from build123d import *

# Parameters (mm, degrees)
SKETCH1_R               = 1.5
BOSS_EXTRUDE1_DEPTH     = 3.5
SKETCH2_R               = 6.4
BOSS_EXTRUDE2_DEPTH     = 25
SKETCH3_R               = 2.8
CUT_EXTRUDE1_DEPTH      = 29.5
SKETCH6_R               = 9.569614172
CUT_EXTRUDE6_DEPTH      = 7.5
SKETCH7_R               = 17.775779512
SKETCH7_R_2             = 6.25
CUT_EXTRUDE7_DEPTH      = 7.5
SKETCH8_R               = 1
CUT_EXTRUDE8_DEPTH      = 4.5
SKETCH9_R               = 2
CUT_EXTRUDE9_DEPTH      = 13
CUT_EXTRUDE9_DEPTH_BACK = 1


with BuildPart() as part:
    # Sketch1 → Boss-Extrude1 (new body)
    with BuildSketch(Plane.XY):
        with BuildLine():
            Line((-14.730127019, -3.5044428), (-4.330127019, 14.508885599))
            ThreePointArc((-4.330127019, 14.508885599), (0, 17.008885599), (4.330127019, 14.508885599))
            Line((4.330127019, 14.508885599), (14.730127019, -3.5044428))
            ThreePointArc((14.730127019, -3.5044428), (14.730127019, -8.5044428), (10.4, -11.0044428))
            Line((10.4, -11.0044428), (-10.4, -11.0044428))
            ThreePointArc((-10.4, -11.0044428), (-14.730127019, -8.5044428), (-14.730127019, -3.5044428))
        make_face()
        with Locations((0, 12.008885599)):
            Circle(SKETCH1_R, mode=Mode.SUBTRACT)
        with Locations((-10.4, -6.0044428)):
            Circle(SKETCH1_R, mode=Mode.SUBTRACT)
        with Locations((10.4, -6.0044428)):
            Circle(SKETCH1_R, mode=Mode.SUBTRACT)
    extrude(amount=BOSS_EXTRUDE1_DEPTH)

    # Sketch2 → Boss-Extrude2 (add)
    with BuildSketch(Plane.XY.offset(3.5)):
        Circle(SKETCH2_R)
    extrude(amount=BOSS_EXTRUDE2_DEPTH)

    # Sketch3 → Cut-Extrude1 (cut, through all)
    with BuildSketch(Plane.XY.offset(28.5)):
        Circle(SKETCH3_R)
    extrude(amount=-CUT_EXTRUDE1_DEPTH, mode=Mode.SUBTRACT)

    # Sketch6 → Cut-Extrude6 (cut)
    with BuildSketch(Plane.XY.offset(26.5)):
        Circle(SKETCH6_R)
        Polygon((7, 0), (4.452808103, 0.65), (4.435733208, 0.757806641), (6.657395614, 2.163118961), (4.034011116, 1.994180112), (3.984457842, 2.091433888), (5.663118961, 4.114496766), (3.220337014, 3.14315598), (3.14315598, 3.220337014), (4.114496766, 5.663118961), (2.091433888, 3.984457842), (1.994180112, 4.034011116), (2.163118961, 6.657395614), (0.757806641, 4.435733208), (0.65, 4.452808103), (0, 7), (-0.65, 4.452808103), (-0.757806641, 4.435733208), (-2.163118961, 6.657395614), (-1.994180112, 4.034011116), (-2.091433888, 3.984457842), (-4.114496766, 5.663118961), (-3.14315598, 3.220337014), (-3.220337014, 3.14315598), (-5.663118961, 4.114496766), (-3.984457842, 2.091433888), (-4.034011116, 1.994180112), (-6.657395614, 2.163118961), (-4.435733208, 0.757806641), (-4.452808103, 0.65), (-7, 0), (-4.452808103, -0.65), (-4.435733208, -0.757806641), (-6.657395614, -2.163118961), (-4.034011116, -1.994180112), (-3.984457842, -2.091433888), (-5.663118961, -4.114496766), (-3.220337014, -3.14315598), (-3.14315598, -3.220337014), (-4.114496766, -5.663118961), (-2.091433888, -3.984457842), (-1.994180112, -4.034011116), (-2.163118961, -6.657395614), (-0.757806641, -4.435733208), (-0.65, -4.452808103), (0, -7), (0.65, -4.452808103), (0.757806641, -4.435733208), (2.163118961, -6.657395614), (1.994180112, -4.034011116), (2.091433888, -3.984457842), (4.114496766, -5.663118961), (3.14315598, -3.220337014), (3.220337014, -3.14315598), (5.663118961, -4.114496766), (3.984457842, -2.091433888), (4.034011116, -1.994180112), (6.657395614, -2.163118961), (4.435733208, -0.757806641), (4.452808103, -0.65), align=None, mode=Mode.SUBTRACT)
    extrude(amount=-CUT_EXTRUDE6_DEPTH, mode=Mode.SUBTRACT)

    # Sketch7 → Cut-Extrude7 (cut)
    with BuildSketch(Plane.XY.offset(26.5)):
        Circle(SKETCH7_R)
        Circle(SKETCH7_R_2, mode=Mode.SUBTRACT)
    extrude(amount=-CUT_EXTRUDE7_DEPTH, mode=Mode.SUBTRACT)

    # Sketch8 → Cut-Extrude8 (cut, through all)
    with BuildSketch(Plane.XY.offset(3.5)):
        with Locations((8.229165125, 4.7511107)):
            Circle(SKETCH8_R)
        with Locations((0, -9.5022214)):
            Circle(SKETCH8_R)
        with Locations((-8.229165125, 4.7511107)):
            Circle(SKETCH8_R)
    extrude(amount=-CUT_EXTRUDE8_DEPTH, mode=Mode.SUBTRACT)

    # Sketch9 → Cut-Extrude9 (cut, two sides)
    with BuildSketch(Plane.XY.offset(3.5)) as cut_extrude9_sk:
        with Locations((8.229165125, 4.7511107)):
            Circle(SKETCH9_R)
        with Locations((0, -9.5022214)):
            Circle(SKETCH9_R)
        with Locations((-8.229165125, 4.7511107)):
            Circle(SKETCH9_R)
    extrude(amount=CUT_EXTRUDE9_DEPTH, mode=Mode.SUBTRACT)
    extrude(cut_extrude9_sk.sketch, amount=-CUT_EXTRUDE9_DEPTH_BACK, mode=Mode.SUBTRACT)


solid = part.part
Design review of the part built by this model. Coordinates are the model's own, in mm. A direction names the side the tool comes from. Give positions to 0.01 mm unless a question says otherwise; leave off trailing zeros. Order: outer loops, then holes, each group sorted by start corner. A loop starts at its lowest first (then second) coordinate and runs counter-clockwise, first axis right, second up.
1. For pin 1 Ø3 at (x, y) = (8.23, 4.75) entering from +Z; pin 2 Ø4.5 at (x, y) = (8.23, 4.75) entering from +Z; pin 3 Ø4 at (x, z) = (-2.5, 14) entering from -Y, all flat-tipped, find the tip position at first contact; note any pin that passes through.
Solution:
pin 1: stops at z = 2.5
pin 2: stops at z = 3.5
pin 3: stops at y = -6.38
2. To check wall thickness, follow L1, parallel to X at y = 5.5, z = 23.5; L2, parallel to Z at x = -4, y = 4.25; L3, parallel to Z at x = -1.5, y = 11.5. State the ranges of each line that lie inside material, in increasing order.
Solution:
L1: x = -2.09 to -1.43, -0.38 to 0.38, 1.43 to 2.09
L2: z = 0 to 19, 26.5 to 28.5
L3: z = 0 to 3.5
3. Mouldability with a two-part tool opening along Y and no side actions: class faces 5 (the flat face through (-1.246, 5.207, 22.803)), 6 (the flat face through (3, -1, 28.5)), 7 (the flat face through (7, 4, 2.5)) as +Y half, -Y half, draft (parallel to the pull), parting line (faces both ways), or undercut.
Solution:
face 5: +Y half
face 6: draft
face 7: undercut
4. Add section A-A, the plane y = 11.5. State the section outline as (x, z) points.
Solution:
outline: (-6.07, 0) - (-1.41, 0) - (-1.41, 3.5) - (-6.07, 3.5) - close; (1.41, 0) - (6.07, 0) - (6.07, 3.5) - (1.41, 3.5) - close
5. Tool access review of faces 1 (the cylindrical face through (-6.532, 3.693, 3.007)), 2 (the flat face through (5.337, -0.424, 22.803)), 3 (the flat face through (0.424, 5.337, 22.803)), 4 (the flat face through (4.971, 2.055, 22.803)): name each direction out of +Z, -Z, +X, -X, +Y, -Y from which nothing blocks a thin tool from reaching the whole face with its end or side.
Solution:
face 1: +Z
face 2: +X
face 3: +Y
face 4: none
6. Add section B-B, the plane z = 14.75. State the section outline as (x, y) points, then the cut area to 3 significant figures.
Solution:
outline: circle Ø12.8 at (0, 0); hole circle Ø5.6 at (0, 0)
area: 104 mm2
